```python
from build123d import *

# Parameters (mm, degrees)
EXTRUDE_1_DEPTH     = 8
SKETCH_2_R          = 37.5
SKETCH_2_R_2        = 1.5
EXTRUDE_2_DEPTH     = 10
SKETCH_3_R          = 20
EXTRUDE_3_DEPTH     = 15.5
SKETCH_4_R          = 12.5
CUT_EXTRUDE_1_DEPTH = 63.727585638
SKETCH_5_R          = 7.5
CUT_EXTRUDE_2_DEPTH = 4
FILLET_1_R          = 4
SKETCH_6_R          = 1.5
CUT_EXTRUDE_3_DEPTH = 5.5
SKETCH_9_R          = 1.5
CUT_EXTRUDE_4_DEPTH = 30
SKETCH_10_R         = 1.5
CUT_EXTRUDE_5_DEPTH = 25.5


with BuildPart() as part:
    # 草图1 → 凸台-拉伸1 (new body)
    with BuildSketch(Plane(origin=(0, 0, 0), x_dir=(1, 0, 0), z_dir=(0, 1, 0))):
        with BuildLine():
            Line((-20, 0), (-20, 31.721443851))
            ThreePointArc((-20, 31.721443851), (0, 37.5), (20, 31.721443851))
            Line((20, 31.721443851), (20, 0))
            ThreePointArc((20, 0), (0, -20), (-20, 0))
        make_face()
    extrude(amount=EXTRUDE_1_DEPTH)

    # 草图2 → 凸台-拉伸2 (add)
    with BuildSketch(Plane(origin=(0, 8, 0), x_dir=(1, 0, 0), z_dir=(0, 1, 0))):
        with Locations(Location((0, 0, 0), (0, 0, 122.230952636))):
            Circle(SKETCH_2_R)
        with Locations(Location((0, -31.5, 0), (0, 0, 270))):
            Circle(SKETCH_2_R_2, mode=Mode.SUBTRACT)
    extrude(amount=EXTRUDE_2_DEPTH)

    # 草图3 → 凸台-拉伸3 (add)
    with BuildSketch(Plane(origin=(0, 18, 0), x_dir=(1, 0, 0), z_dir=(0, 1, 0))):
        with Locations(Location((0, 0, 0), (0, 0, 270))):
            Circle(SKETCH_3_R)
    extrude(amount=EXTRUDE_3_DEPTH)

    # 草图4 → 切除-拉伸1 (cut, through all)
    with BuildSketch(Plane(origin=(0, 33.5, 0), x_dir=(1, 0, 0), z_dir=(0, 1, 0))):
        with Locations(Location((0, 0, 0), (0, 0, 270))):
            Circle(SKETCH_4_R)
    extrude(amount=-CUT_EXTRUDE_1_DEPTH, mode=Mode.SUBTRACT)

    # 草图5 → 切除-拉伸2 (cut)
    with BuildSketch(Plane.XZ):
        with Locations(Location((0, -28.5, 0), (0, 0, 270))):
            Circle(SKETCH_5_R)
    extrude(amount=-CUT_EXTRUDE_2_DEPTH, mode=Mode.SUBTRACT)

    # 圆角1
    fillet_1_edges = [part.edges().sort_by_distance(p)[0] for p in [
        (0, 4, -21),
    ]]
    fillet(fillet_1_edges, radius=FILLET_1_R - 0.0001)  # a hair under: the kernel refuses the full size

    # 草图6 → 切除-拉伸3 (cut)
    with BuildSketch(Plane.XZ.offset(-4)):
        with Locations(Location((0, -28.5, 0), (0, 0, 270))):
            Circle(SKETCH_6_R)
    extrude(amount=-CUT_EXTRUDE_3_DEPTH, mode=Mode.SUBTRACT)

    # 草图9 → 切除-拉伸4 (cut)
    with BuildSketch(Plane.XY):
        with Locations((0, 8)):
            Circle(SKETCH_9_R)
    extrude(amount=-CUT_EXTRUDE_4_DEPTH, mode=Mode.SUBTRACT)

    # 草图10 → 切除-拉伸5 (cut)
    with BuildSketch(Plane(origin=(0, 33.5, 0), x_dir=(1, 0, 0), z_dir=(0, 1, 0))):
        with Locations(Location((0, 16.5, 0), (0, 0, 270))):
            Circle(SKETCH_10_R)
    extrude(amount=-CUT_EXTRUDE_5_DEPTH, mode=Mode.SUBTRACT)


solid = part.part
```
Here's how the part is built. I have some questions about the finished solid (model axes, mm). A direction names the side the tool comes from. Coordinates: 2 decimals unless noted, no trailing zeros. Order: outer loops, then holes, each group sorted by start corner. A loop starts at its lowest first (then second) coordinate and runs counter-clockwise, first axis right, second up. Notation, with made-up numbers: (-20.75, 87.25) -> (28.25, 87.25) arc R27 cw to (28.25, 124.25) -> close; hole circle Ø3 at (39.25, 43.5). An arc over 180 degrees is marked (long way). Return JSON: item names as keys, results as strings.
1) If we section it at C-C on z = 18.5: List the corners of the cut face in (x, y) for me, plus the area to 3 significant figures.
Conclusion:
{"outline": "(-32.62, 8) -> (-7.6, 8) -> (-7.6, 0) -> (7.6, 0) -> (7.6, 8) -> (32.62, 8) -> (32.62, 18) -> (7.6, 18) -> (7.6, 33.5) -> (-7.6, 33.5) -> (-7.6, 18) -> (-32.62, 18) -> close", "area": "1,010 mm²"}
2) I'm going to push flat-ended pins straight in: P1, Ø5, axis at y = 15, z = 8.5, coming from the +X side; P2, Ø2, axis at y = 28.5, z = 22.5, coming from the -X side; P3, Ø12, axis at x = -11.5, y = 16.5, coming from the -Z side; P4, Ø9, axis at y = 4, z = -10, coming from the +X side. Where does each tip first touch, or does it pass through?
Conclusion:
{"P1": "stops at x = 37.02", "P2": "passes through", "P3": "stops at z = -37.09", "P4": "stops at x = 36.65"}
3) If I drill on probe 1 along X at (y, z) = (25, 0); probe 2 along X at (y, z) = (5, -10); probe 3 along Z at (x, y) = (-2, 10), over which ranges is the centre line in solid material (lowest first)?
Conclusion:
{"probe 1": "x = -20 to -12.5, 12.5 to 20", "probe 2": "x = -20 to -7.5, 7.5 to 20", "probe 3": "z = -37.45 to -12.34, 12.34 to 37.45"}
4) If we section it at D-D on y = 11.5: List the corners of the cut face in (x, z) for me.
Conclusion:
{"outline": "circle Ø75 at (0, 0); hole circle Ø25 at (0, 0); hole circle Ø3 at (0, -16.5); hole circle Ø3 at (0, 31.5)"}
5) Thinking about a two-plate mould opening in X: for faces 5 (the cylindrical face through (1.487, 5.528, -28.305)), 6 (the cylindrical face through (0, 21, -18)), 7 (the cylindrical face through (-19.524, 25.642, -4.336)), 8 (the flat face through (9, 33.5, 9)), which applies, +X half, -X half, draft (parallel to the pull), parting line (faces both ways), or undercut?
Conclusion:
{"face 5": "undercut", "face 6": "undercut", "face 7": "parting line", "face 8": "draft"}
6) If we section it at A-A on z = 31.5: List the corners of the cut face in (x, y) for me.
Conclusion:
{"outline": "(-20.35, 8) -> (-1.5, 8) -> (-1.5, 18) -> (-20.35, 18) -> close; (1.5, 8) -> (20.35, 8) -> (20.35, 18) -> (1.5, 18) -> close"}
7) On a 3-axis mill with a long thin cutter (end or side, diameter ignored), from which of +Z, -Z, +X, -X, +Y, -Y can I reach the whole of each face in a straight line? I mean faces 1 (the flat face through (20, 4, -16)), 2 (the flat face through (5, 18, -22)), 3 (the flat face through (-5, 8, 24)), 4 (the flat face through (0, 9.5, -28)). Say none if no direction works.
Conclusion:
{"face 1": "+Z, -Z, +X, -Y", "face 2": "+Y", "face 3": "+Z, -Y", "face 4": "-Y"}
8) If we section it at B-B on y = 5: List the corners of the cut face in (x, z) for me, plus the area to 3 significant figures.
Conclusion:
{"outline": "(-20, -31.72) arc R37.5 ccw to (20, -31.72) -> (20, 0) arc R20 ccw to (-20, 0) -> close; hole circle Ø25 at (0, 0); hole circle Ø3 at (0, -28.5)", "area": "1,560 mm²"}
